from build123d import *

# Parameters (mm, degrees)
SKETCH2_W                = 10
SKETCH2_H                = 86
BOSS_EXTRUDE1_DEPTH      = 10
SKETCH3_W                = 10
SKETCH3_H                = 86
BOSS_EXTRUDE2_DEPTH      = 23
BOSS_EXTRUDE3_REACH      = 246.16
BOSS_EXTRUDE4_DEPTH      = 100
BOSS_EXTRUDE4_DEPTH_BACK = 5
SKETCH5_R                = 47.55
SKETCH7_W                = 10
SKETCH7_H                = 18.447060317
BOSS_EXTRUDE6_DEPTH      = 30
CUT_EXTRUDE2_DEPTH       = 10
BOSS_EXTRUDE7_REACH      = 275.742
SKETCH6_R                = 45.55
CUT_EXTRUDE1_DEPTH       = 100
SKETCH10_W               = 15
SKETCH10_H               = 10
SKETCH10_W_2             = 10
SKETCH10_H_2             = 15
BOSS_EXTRUDE8_DEPTH      = 28.5
FILLET1_R                = 30
FILLET2_R                = 30
FILLET3_R                = 30
SKETCH11_W               = 250
SKETCH11_H               = 33
CUT_EXTRUDE3_DEPTH       = 234.52646531


with BuildPart() as part:
    # Sketch2 → Boss-Extrude1 (new body)
    with BuildSketch(Plane(origin=(0, 0, 0), x_dir=(1, 0, 0), z_dir=(0, 1, 0))):
        Polygon((-125, -75), (-115, -75), (-115, -48), (-47, -48), (-47, -75), (47, -75), (47, -48), (115, -48), (115, -75), (125, -75), (125, 75), (115, 75), (115, 48), (47, 48), (47, 75), (-47, 75), (-47, 48), (-115, 48), (-115, 75), (-125, 75), align=None)
        with Locations((-110, 0)):
            Rectangle(SKETCH2_W, SKETCH2_H, mode=Mode.SUBTRACT)
    extrude(amount=BOSS_EXTRUDE1_DEPTH)

    # Sketch3 → Boss-Extrude2 (add)
    with BuildSketch(Plane(origin=(0, 10, 0), x_dir=(1, 0, 0), z_dir=(0, 1, 0))):
        Polygon((-47, 48), (-47, 75), (47, 75), (47, 48), (26, 48), (26, 27), (93, 27), (93, 48), (115, 48), (115, 75), (125, 75), (125, -75), (115, -75), (115, -48), (93, -48), (93, -27), (26, -27), (26, -48), (47, -48), (47, -75), (-47, -75), (-47, -48), (-26, -48), (-26, -27), (-93, -27), (-93, -48), (-115, -48), (-115, -75), (-125, -75), (-125, 75), (-115, 75), (-115, 48), (-93, 48), (-93, 27), (-26, 27), (-26, 48), align=None)
        with Locations((-110, 0)):
            Rectangle(SKETCH3_W, SKETCH3_H, mode=Mode.SUBTRACT)
    extrude(amount=BOSS_EXTRUDE2_DEPTH)

    # Sketch4 → Boss-Extrude3 (add, up to next)
    with BuildSketch(Plane.ZY.offset(105), mode=Mode.PRIVATE) as boss_extrude3_sk1:
        Polygon((-43, 0), (-9.223530158, 14.703891082), (-43, 33), align=None)
    boss_extrude3_tool1 = extrude(boss_extrude3_sk1.sketch, amount=BOSS_EXTRUDE3_REACH, mode=Mode.PRIVATE) - part.part
    # Sketch4 → Boss-Extrude3 (add, up to next)
    with BuildSketch(Plane.ZY.offset(105), mode=Mode.PRIVATE) as boss_extrude3_sk2:
        Polygon((43, 0), (9.223530158, 14.703891082), (-24.552939683, 33), (43, 33), align=None)
    boss_extrude3_tool2 = extrude(boss_extrude3_sk2.sketch, amount=BOSS_EXTRUDE3_REACH, mode=Mode.PRIVATE) - part.part
    add(boss_extrude3_tool1.solids().sort_by_distance((-105, 15.901297, -31.741177))[0])
    add(boss_extrude3_tool2.solids().sort_by_distance((-105, 21.685197, 19.901194))[0])



with BuildPart() as body_2:
    # Sketch5 → Boss-Extrude4 (new, two sides: drawn at the far end of the back side and taken through both)
    with BuildSketch(Plane(origin=(-115, 0, 0), x_dir=(0, 0, -1), z_dir=(1, 0, 0)).offset(-BOSS_EXTRUDE4_DEPTH_BACK)):
        with Locations((0, 80.55)):
            Circle(SKETCH5_R)
    extrude(amount=BOSS_EXTRUDE4_DEPTH + BOSS_EXTRUDE4_DEPTH_BACK)


with BuildPart() as part_1:
    add(part.part)

    add(body_2.part)  # Boss-Extrude6 merges body 2
    # Sketch7 → Boss-Extrude6 (add)
    with BuildSketch(Plane(origin=(0, 33, 0), x_dir=(1, 0, 0), z_dir=(0, 1, 0))):
        Polygon((-120, 0), (-120, 48), (-93, 48), (-93, 27), (-15, 27), (-15, -27), (-93, -27), (-93, -48), (-120, -48), align=None)
        with Locations((-110, 33.776469842)):
            Rectangle(SKETCH7_W, SKETCH7_H, mode=Mode.SUBTRACT)
    extrude(amount=BOSS_EXTRUDE6_DEPTH)

    # Sketch8 → Cut-Extrude2 (cut)
    with BuildSketch(Plane.ZY.offset(105)):
        Polygon((-43, 46.626077643), (-41.871641374, 62.212018017), (-24.552939683, 62.212018017), (-24.552939683, 33), (-43, 33), align=None)
    extrude(amount=CUT_EXTRUDE2_DEPTH, mode=Mode.SUBTRACT)

    # Sketch9 → Boss-Extrude7 (add, up to next)
    with BuildSketch(Plane.ZY.offset(105), mode=Mode.PRIVATE) as boss_extrude7_sk1:
        Polygon((-42.138917347, 58.520153318), (-43, 46.626077643), (-43, 62.212018017), (-41.871641374, 62.212018017), align=None)
    boss_extrude7_tool1 = extrude(boss_extrude7_sk1.sketch, amount=BOSS_EXTRUDE7_REACH, mode=Mode.PRIVATE) - part_1.part
    add(boss_extrude7_tool1.solids().sort_by_distance((-105, 57.016705, -42.62388))[0])

    # Sketch6 → Cut-Extrude1 (cut)
    with BuildSketch(Plane(origin=(-15, 0, 0), x_dir=(0, 0, -1), z_dir=(1, 0, 0))):
        with Locations((0, 80.55)):
            Circle(SKETCH6_R)
    extrude(amount=-CUT_EXTRUDE1_DEPTH, mode=Mode.SUBTRACT)

    # Sketch10 → Boss-Extrude8 (add)
    with BuildSketch(Plane(origin=(0, 33, 0), x_dir=(1, 0, 0), z_dir=(0, 1, 0))):
        with Locations((12.5, 39)):
            Rectangle(SKETCH10_W, SKETCH10_H)
        with Locations((12.5, -39)):
            Rectangle(SKETCH10_W, SKETCH10_H)
        with Locations((63, 0)):
            Rectangle(SKETCH10_W_2, SKETCH10_H_2)
    extrude(amount=BOSS_EXTRUDE8_DEPTH)

    # Fillet1
    # the kernel refuses this fillet: 30 mm, written as the material it adds along each edge
    with BuildSketch(Plane(origin=(5, 33, 44), x_dir=(0, 0, 1), z_dir=(1, 0, 0))) as fillet1_piece_1:
        with BuildLine():
            CenterArc((29.962476533, -30), FILLET1_R, 90, 87.134016017)
            Line((0, -28.5), (0, 0))
            Line((0, 0), (29.962476533, 0))
        make_face()
    extrude(amount=15)

    # Fillet2
    # the kernel refuses this fillet: 30 mm, written as the material it adds along each edge
    with BuildSketch(Plane(origin=(20, 33, -44), x_dir=(0, 0, -1), z_dir=(-1, 0, 0))) as fillet2_piece_1:
        with BuildLine():
            CenterArc((29.962476533, -30), FILLET2_R, 90, 87.134016017)
            Line((0, -28.5), (0, 0))
            Line((0, 0), (29.962476533, 0))
        make_face()
    extrude(amount=15)

    # Fillet3
    # the kernel refuses this fillet: 30 mm, written as the material it adds along each edge
    with BuildSketch(Plane(origin=(68, 33, 7.5), x_dir=(1, 0, 0), z_dir=(0, 0, -1))) as fillet3_piece_1:
        with BuildLine():
            CenterArc((29.962476533, -30), FILLET3_R, 90, 87.134016017)
            Line((0, -28.5), (0, 0))
            Line((0, 0), (29.962476533, 0))
        make_face()
    extrude(amount=15)

    # Sketch11 → Cut-Extrude3 (cut, through all)
    with BuildSketch(Plane.XY.offset(75)):
        with Locations((0, 16.5)):
            Rectangle(SKETCH11_W, SKETCH11_H)
    extrude(amount=-CUT_EXTRUDE3_DEPTH, mode=Mode.SUBTRACT)


with BuildPart() as cut_extrude3_piece_1:
    # of the separate pieces the step leaves, piece 1, a body of its own (cut_extrude3_pieces)
    add(part_1.part.solids().sort_by_distance((-93, 33, 27))[0])


with BuildPart() as cut_extrude3_piece_2:
    # of the separate pieces the step leaves, piece 2, a body of its own (cut_extrude3_pieces)
    add(part_1.part.solids().sort_by_distance((97.962476533, 33, 7.5))[0])


with BuildPart() as cut_extrude3_piece_3:
    # of the separate pieces the step leaves, piece 3, a body of its own (cut_extrude3_pieces)
    add(part_1.part.solids().sort_by_distance((20, 33, 34))[0])


with BuildPart() as cut_extrude3_piece_4:
    # of the separate pieces the step leaves, piece 4, a body of its own (cut_extrude3_pieces)
    add(part_1.part.solids().sort_by_distance((20, 33, -73.962476533))[0])


solid = cut_extrude3_piece_1.part
Here's how the part is built. I have some questions about the finished solid (model axes, mm). A direction names the side the tool comes from. Give positions to 0.01 mm unless a question says otherwise; leave off trailing zeros. Order: outer loops, then holes, each group sorted by start corner. A loop starts at its lowest first (then second) coordinate and runs counter-clockwise, first axis right, second up. Notation, with made-up numbers: (-2.5, 18.5) -> (53.5, 18.5) arc R20 cw to (53.5, 22.5) -> close; hole circle Ø11 at (-31, 43). An arc over 180 degrees is marked (long way). One line per item, written item: value. Start each with the question number.
1. Imagine slicing it at B-B, the plane z = -38.5. List the corners of the cut face in (x, y) for me, plus the area to 3 significant figures.
2. I need wall thicknesses on probe 1 along Y at (x, z) = (-41.5, 0); probe 2 along X at (y, z) = (47, -39); probe 3 along X at (y, z) = (79.5, 44.5). Which ranges of each line are inside material? Lowest first, please. Write a range as from..to.
3. For faces 4 (the face through (-53, 37, 27)), 5 (the face through (-55, 37, -27)), 6 (the face through (-110, 40, -43)), which set-ups out of +Z, -Z, +X, -X, +Y, -Y let a thin tool reach every point of the face, with its end or its side?
4. Imagine slicing it at C-C, the plane z = 0. List the corners of the cut face in (x, y) for me.
5. We'd pull the mould along X, two halves only. Please class faces 1 (the face through (-93, 44, 40)), 2 (the face through (-110, 38, -24.553)), 3 (the face through (-64.3, 52.834, 36.147)): released by +X, released by -X, zero draft, split by the parting line, or undercut.
6. Imagine slicing it at D-D, the plane y = 80.55. List the corners of the cut face in (x, z) for me.
7. Imagine slicing it at A-A, the plane x = -102.5. List the corners of the cut face in (y, z) for me.
8. Will these pins go through, and if not, where does the flat tip stop? pin 1 Ø10.5 at (y, z) = (45, -40) entering from +X; pin 2 Ø1.5 at (x, z) = (-50.5, -22.5) entering from +Y; pin 3 Ø6.5 at (y, z) = (42.5, 33.5) entering from +X; pin 4 Ø12 at (x, y) = (-48, 77.5) entering from +Z.
Values follow:
1. outline: (-120, 33) -> (-115, 33) -> (-115, 104.89) -> (-15, 104.89) -> (-15, 108.46) -> (-120, 108.46) -> close; (-105, 33) -> (-93, 33) -> (-93, 52.64) -> (-15, 52.64) -> (-15, 56.21) -> (-105, 56.21) -> close
1. area: 1,290 mm2
2. probe 1: y = 33..35, 126.1..128.1
2. probe 2: x = -120..-115, -105..-93
2. probe 3: x = -120..-115
3. face 4: +Z, +X, -Y
3. face 5: -Z, +X, -Y
3. face 6: -Y
4. outline: (-120, 33) -> (-15, 33) -> (-15, 35) -> (-115, 35) -> (-115, 126.1) -> (-15, 126.1) -> (-15, 128.1) -> (-120, 128.1) -> close
5. face 1: released by +X
5. face 2: undercut
5. face 3: zero draft
6. outline: (-120, -47.55) -> (-15, -47.55) -> (-15, -45.55) -> (-115, -45.55) -> (-115, 45.55) -> (-15, 45.55) -> (-15, 47.55) -> (-120, 47.55) -> close
7. outline: (33, -48) -> (63, -48) -> (63, -44.19) arc R47.55 ccw (long way) to (63, 44.19) -> (63, 48) -> (33, 48) -> close; hole circle Ø91.1 at (80.55, 0)
8. pin 1: stops at x = -93
8. pin 2: stops at y = 122.83
8. pin 3: stops at x = -15
8. pin 4: stops at z = 47.55
